Geometry: final body of the model. Coordinates: model frame, mm. Face numbers are marked on the shaded views. A direction names the side the tool comes from. Give positions to 0.01 mm unless a question says otherwise; leave off trailing zeros. Write each loop counter-clockwise with the first axis right and the second up, starting at its lowest first coordinate (ties: lowest second). Pieces come first, ordered by that corner, then holes. Notation, with made-up numbers: (86.25, 33.5) - (121.25, 33.5) arc R16 cw to (121.25, 51.5) - close; hole circle Ø8 at (-22.5, -30.75). An arc over 180 degrees is marked (long way). Return JSON: item names as keys, results as strings.
from build123d import *

# Parameters (mm, degrees)
SKETCH_1_W          = 15
SKETCH_1_H          = 15
EXTRUDE_1_DEPTH     = 60
SKETCH_4_W          = 15
SKETCH_4_H          = 44
EXTRUDE_4_DEPTH     = 20
SKETCH_5_W          = 15
SKETCH_5_H          = 44
EXTRUDE_5_DEPTH     = 20
SKETCH_6_W          = 10
SKETCH_6_H          = 10
CUT_EXTRUDE_1_DEPTH = 70
SKETCH_7_W          = 10
SKETCH_7_H          = 10
CUT_EXTRUDE_2_DEPTH = 70


with BuildPart() as part:
    # 草图1 → 凸台-拉伸1 (new body)
    with BuildSketch(Plane(origin=(0, 0, 0), x_dir=(1, 0, 0), z_dir=(0, 1, 0))):
        Rectangle(SKETCH_1_W, SKETCH_1_H)
    extrude(amount=EXTRUDE_1_DEPTH)

    # 草图4 → 凸台-拉伸4 (add)
    with BuildSketch(Plane.XY.offset(7.5)):
        with Locations((0, 38)):
            Rectangle(SKETCH_4_W, SKETCH_4_H)
    extrude(amount=EXTRUDE_4_DEPTH)

    # 草图5 → 凸台-拉伸5 (add)
    with BuildSketch(Plane(origin=(7.5, 0, 0), x_dir=(0, 0, -1), z_dir=(1, 0, 0))):
        with Locations((0, 38)):
            Rectangle(SKETCH_5_W, SKETCH_5_H)
    extrude(amount=EXTRUDE_5_DEPTH)

    # 草图6 → 切除-拉伸1 (cut)
    with BuildSketch(Plane.XY.offset(27.5)):
        with Locations((0, 52)):
            Rectangle(SKETCH_6_W, SKETCH_6_H)
        with Locations((0, 24)):
            Rectangle(SKETCH_6_W, SKETCH_6_H)
    extrude(amount=-CUT_EXTRUDE_1_DEPTH, mode=Mode.SUBTRACT)

    # 草图7 → 切除-拉伸2 (cut)
    with BuildSketch(Plane(origin=(27.5, 0, 0), x_dir=(0, 0, -1), z_dir=(1, 0, 0))):
        with Locations((0, 52)):
            Rectangle(SKETCH_7_W, SKETCH_7_H)
        with Locations((0, 24)):
            Rectangle(SKETCH_7_W, SKETCH_7_H)
    extrude(amount=-CUT_EXTRUDE_2_DEPTH, mode=Mode.SUBTRACT)


solid = part.part
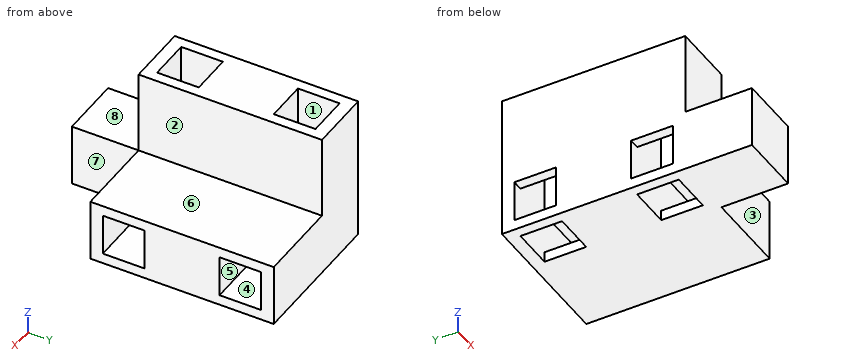
Q1. Section query D-D, the plane z = 20. Return the cut outline in (x, y), plus the area to 3 significant figures.
Answer key:
{"outline": "(-7.5, 16) - (7.5, 16) - (7.5, 60) - (-7.5, 60) - close; hole (-5, 19) - (5, 19) - (5, 29) - (-5, 29) - close; hole (-5, 47) - (5, 47) - (5, 57) - (-5, 57) - close", "area": "460 mm^2"}
Q2. Material intervals for probe 1 along Y at (x, z) = (11, 0); probe 2 along Y at (x, z) = (4, -4); probe 3 along X at (y, z) = (25, 12.5), sorted ascending. Write a range as [from, to].
Answer key:
{"probe 1": "y = [16, 19], [29, 47], [57, 60]", "probe 2": "y = [0, 19], [29, 47], [57, 60]", "probe 3": "x = [-7.5, -5], [5, 7.5]"}
Q3. Set-up query: the marked faces 4, 5, 6, 7 and 8. Return all of +Z, -Z, +X, -X, +Y, -Y with unobstructed straight access to the full face (end or side cutting, diameter ignored); none if empty.
Answer key:
{"face 4": "+X, -X", "face 5": "none", "face 6": "+Z, +X, +Y, -Y", "face 7": "+Z, -Z, +X, -Y", "face 8": "+Z, +X, -X, -Y"}
Q4. Section query A-A, the plane x = -3.5. Return the cut outline in (y, z), plus the area to 3 significant figures.
Answer key:
{"outline": "(0, -7.5) - (19, -7.5) - (19, 27.5) - (16, 27.5) - (16, 7.5) - (0, 7.5) - close; (29, -7.5) - (47, -7.5) - (47, 27.5) - (29, 27.5) - close; (57, -7.5) - (60, -7.5) - (60, 27.5) - (57, 27.5) - close", "area": "1,080 mm^2"}
Q5. Section query B-B, the plane z = 2. Return the cut outline in (x, y).
Answer key:
{"outline": "(-7.5, 0) - (7.5, 0) - (7.5, 16) - (27.5, 16) - (27.5, 19) - (-7.5, 19) - close; (-7.5, 29) - (27.5, 29) - (27.5, 47) - (-7.5, 47) - close; (-7.5, 57) - (27.5, 57) - (27.5, 60) - (-7.5, 60) - close"}
Q6. Mould query, pull axis X, two halves, no side actions, for the marked faces 1, 2 and 3. Classes: pulls with the +X half, pulls with the -X half, needs draft (parallel to the pull), parting line crosses it, or undercut.
Answer key:
{"face 1": "undercut", "face 2": "pulls with the +X half", "face 3": "needs draft"}
Q7. Pin query (flat end, axial travel): P1, Ø11, axis at y = 53, z = 15, coming from the +X side; P2, Ø1, axis at y = 14, z = 12, coming from the -X side; P3, Ø3, axis at x = 16, y = 23, coming from the +Z side; P4, Ø4, axis at x = 22, z = 1.5, coming from the -Y side. Return the tip coordinate at first contact, or that it passes through.
Answer key:
{"P1": "stops at x = 7.5", "P2": "passes through", "P3": "stops at z = 7.5", "P4": "stops at y = 16"}
Q8. Section query C-C, the plane y = 53. Return the cut outline in (x, z), plus the area to 3 significant figures.
Answer key:
{"outline": "(-7.5, -7.5) - (-5, -7.5) - (-5, -5) - (-7.5, -5) - close; (-7.5, 5) - (-5, 5) - (-5, 27.5) - (-7.5, 27.5) - close; (5, -7.5) - (27.5, -7.5) - (27.5, -5) - (5, -5) - close; (5, 5) - (27.5, 5) - (27.5, 7.5) - (7.5, 7.5) - (7.5, 27.5) - (5, 27.5) - close", "area": "225 mm^2"}
